Work out the finished part from the listing and answer in its coordinate system (mm). A direction names the side the tool comes from. Round coordinates to 2 decimals unless told otherwise and drop trailing zeros. Order: outer loops, then holes, each group sorted by start corner. A loop starts at its lowest first (then second) coordinate and runs counter-clockwise, first axis right, second up.
from build123d import *

# Parameters (mm, degrees)
SKETCH_2_W           = 30.5
SKETCH_2_H           = 20.5
SKETCH_2_W_2         = 22.5
SKETCH_2_H_2         = 12.5
EXTRUDE_1_DEPTH      = 12
SKETCH_3_W           = 2.75
SKETCH_3_H           = 10
EXTRUDE_2_DEPTH      = 3
SKETCH_4_W           = 4.940698383
SKETCH_4_H           = 10
CUT_EXTRUDE_1_DEPTH  = 9
SKETCH_7_R           = 1.25
CUT_EXTRUDE_2_DEPTH  = 23.584563312
SKETCH_12_W          = 15
SKETCH_12_H          = 20.5
EXTRUDE_5_DEPTH      = 15
SKETCH_13_W          = 10
SKETCH_13_H          = 10
CUT_EXTRUDE_6_DEPTH  = 12
EXTRUDE_7_REACH      = 33.133
SKETCH_15_R          = 1.5
CUT_EXTRUDE_7_DEPTH  = 32.30994251
SKETCH_16_W          = 10.43035396
SKETCH_16_H          = 7
CUT_EXTRUDE_8_DEPTH  = 23
CUT_EXTRUDE_9_REACH  = 36.03
SKETCH_17_W          = 10.8
SKETCH_17_H          = 10.8
CUT_EXTRUDE_10_REACH = 33.31
SKETCH_19_W          = 22.9
SKETCH_19_H          = 13.3
CUT_EXTRUDE_12_DEPTH = 12


with BuildPart() as part:
    # 草图2 → 凸台-拉伸1 (new body)
    with BuildSketch(Plane.XY):
        Rectangle(SKETCH_2_W, SKETCH_2_H)
        Rectangle(SKETCH_2_W_2, SKETCH_2_H_2, mode=Mode.SUBTRACT)
    extrude(amount=EXTRUDE_1_DEPTH)

    # 草图3 → 凸台-拉伸2 (add)
    with BuildSketch(Plane.XY.offset(12)):
        with Locations((-16.625, 0)):
            Rectangle(SKETCH_3_W, SKETCH_3_H)
    extrude_2 = extrude(amount=-EXTRUDE_2_DEPTH)

    # 镜向1: 凸台-拉伸2 across plane
    add(extrude_2.mirror(Plane(origin=(0, 0, 0), x_dir=(0, 0, 1), z_dir=(1, 0, 0))))

    # 草图4 → 切除-拉伸1 (cut)
    with BuildSketch(Plane(origin=(0, 0, 0), x_dir=(-1, 0, 0), z_dir=(0, 0, -1))):
        with Locations((15.220349192, 0)):
            Rectangle(SKETCH_4_W, SKETCH_4_H)
    cut_extrude_1 = extrude(amount=-CUT_EXTRUDE_1_DEPTH, mode=Mode.SUBTRACT)

    # 镜向2: 切除-拉伸1 across plane
    add(cut_extrude_1.mirror(Plane(origin=(0, 0, 0), x_dir=(0, 0, 1), z_dir=(1, 0, 0))), mode=Mode.SUBTRACT)

    # 草图7 → 切除-拉伸2 (cut, through all)
    with BuildSketch(Plane(origin=(0, 0, 9), x_dir=(-1, 0, 0), z_dir=(0, 0, -1))):
        with Locations((15.25, 0)):
            Circle(SKETCH_7_R)
    extrude(amount=-CUT_EXTRUDE_2_DEPTH, mode=Mode.SUBTRACT)

    # 草图12 → 凸台-拉伸5 (add)
    with BuildSketch(Plane(origin=(0, 0, 0), x_dir=(-1, 0, 0), z_dir=(0, 0, -1))):
        Rectangle(SKETCH_12_W, SKETCH_12_H)
    extrude(amount=EXTRUDE_5_DEPTH)

    # 草图13 → 切除-拉伸6 (cut)
    with BuildSketch(Plane(origin=(0, 0, -15), x_dir=(-1, 0, 0), z_dir=(0, 0, -1))):
        Rectangle(SKETCH_13_W, SKETCH_13_H)
    extrude(amount=-CUT_EXTRUDE_6_DEPTH, mode=Mode.SUBTRACT)

    # 凸台-拉伸7: up to this face of the body (flat: up to its plane)
    extrude_7_end = Plane(part.part.faces().sort_by_distance((0, 10.25, 0.860406091))[0])
    # 草图14 → 凸台-拉伸7 (add, up to the picked face)
    with BuildSketch(Plane.XZ.offset(10.25), mode=Mode.PRIVATE) as extrude_7_sk1:
        Polygon((-7.5, -3.75), (-7.5, 0), (-12.905079067, 0), align=None)
    extrude_7_tool1 = split(extrude(extrude_7_sk1.sketch, amount=-EXTRUDE_7_REACH, mode=Mode.PRIVATE), bisect_by=extrude_7_end, keep=Keep.BOTH, mode=Mode.PRIVATE)
    extrude_7 = extrude_7_tool1.solids().sort_by(Axis((-9.301693, -10.25, -1.25), (0, 1, 0)))[0]
    add(extrude_7)

    # 镜向6: 凸台-拉伸7 across plane
    add(extrude_7.mirror(Plane(origin=(0, 0, 0), x_dir=(0, 0, 1), z_dir=(1, 0, 0))))

    # 草图15 → 切除-拉伸7 (cut, through all)
    with BuildSketch(Plane.ZY.offset(7.5)):
        with Locations((-11, 0)):
            Circle(SKETCH_15_R)
    extrude(amount=-CUT_EXTRUDE_7_DEPTH, mode=Mode.SUBTRACT)

    # 草图16 → 切除-拉伸8 (cut)
    with BuildSketch(Plane.XY):
        with Locations((16.46517698, 0)):
            Rectangle(SKETCH_16_W, SKETCH_16_H)
    extrude(amount=CUT_EXTRUDE_8_DEPTH, mode=Mode.SUBTRACT)

    # 草图17 → 切除-拉伸9 (cut, up to next)
    with BuildSketch(Plane(origin=(0, 0, -15), x_dir=(-1, 0, 0), z_dir=(0, 0, -1)), mode=Mode.PRIVATE) as cut_extrude_9_sk1:
        Rectangle(SKETCH_17_W, SKETCH_17_H)
    cut_extrude_9_tool1 = extrude(cut_extrude_9_sk1.sketch, amount=-CUT_EXTRUDE_9_REACH, mode=Mode.PRIVATE) & part.part
    add(cut_extrude_9_tool1.solids().sort_by_distance((0, 0, -15))[0], mode=Mode.SUBTRACT)

    # 草图18 → 切除-拉伸10 (cut, up to next)
    with BuildSketch(Plane.ZY.offset(7.5), mode=Mode.PRIVATE) as cut_extrude_10_sk1:
        Polygon((-9.267949192, 3), (-12.732050808, 3), (-14.464101615, 0), (-12.732050808, -3), (-9.267949192, -3), (-7.535898385, 0), align=None)
    cut_extrude_10_tool1 = extrude(cut_extrude_10_sk1.sketch, amount=-CUT_EXTRUDE_10_REACH, mode=Mode.PRIVATE) & part.part
    add(cut_extrude_10_tool1.solids().sort_by_distance((-7.5, 0, -11))[0], mode=Mode.SUBTRACT)

    # 草图19 → 切除-拉伸12 (cut)
    with BuildSketch(Plane.XY.offset(12)):
        with Locations((-0.2, 0)):
            Rectangle(SKETCH_19_W, SKETCH_19_H)
    extrude(amount=-CUT_EXTRUDE_12_DEPTH, mode=Mode.SUBTRACT)


solid = part.part
Item 1: Given pin 1 (1 mm diameter, centred on y = -7, z = 6, fed in from -X); pin 2 (9 mm diameter, centred on y = 3.5, z = -10.5, fed in from -X); pin 3 (3.5 mm diameter, centred on y = -1, z = 4, fed in from +X), each flat-ended and moving along its own axis, determine where each tip first touches the part or whether it passes through.
Item 2: For a pull along X with two mould halves and no side action, classify faces 5 (the face through (0, -5.4, -8)), 6 (the face through (15.25, -8, 6)), 7 (the face through (-7.5, 0, -7)) as released by +X, released by -X, zero draft, split by the parting line, or undercut.
Item 3: Find the intervals of material crossed by line 1 along X through (y, z) = (4.5, 3.25); line 2 along Y through (x, z) = (3.5, -5.5); line 3 along Y through (x, z) = (6, 9.25), in increasing order.
Item 4: Find section C-C (y = 8.5). Write down the section's boundary in (x, z), plus the area to 3 significant figures.
Item 5: Find section A-A (z = -11). Write down the section's boundary in (x, y).
Item 6: Find section B-B (x = 0.5). Write down the section's boundary in (y, z).
Item 7: A tool of negligible diameter and unlimited length cuts with its end or side. For faces 1 (the face through (-5.4, 0, -6)), 2 (the face through (-6, -3, -11)), 3 (the face through (14, -8, 0)), 4 (the face through (17, -5, 11)), from which of +Z, -Z, +X, -X, +Y, -Y can it reach the whole face along a straight path? Write none if from no direction.
Item 8: Find section D-D (x = -7). Write down the section's boundary in (y, z).
Model answer:
1. pin 1: stops at x = -15.25
1. pin 2: stops at x = -7.5
1. pin 3: stops at x = -11.65
2. face 5: undercut
2. face 6: released by +X
2. face 7: released by -X
3. line 1: x = -12.75 to -11.65, 11.25 to 12.75
3. line 2: y = -10.25 to -5.4, 5.4 to 10.25
3. line 3: y = -10.25 to -6.65, 6.65 to 10.25
4. outline: (-15.25, 0) - (-12.91, 0) - (-7.5, -3.75) - (-7.5, -15) - (7.5, -15) - (7.5, -3.75) - (12.91, 0) - (15.25, 0) - (15.25, 12) - (-15.25, 12) - close
4. area: 611 mm2
5. outline: (-7.5, -10.25) - (7.5, -10.25) - (7.5, -1.5) - (5.4, -1.5) - (5.4, -5.4) - (-5.4, -5.4) - (-5.4, -3) - (-7.5, -3) - close; (-7.5, 3) - (-5.4, 3) - (-5.4, 5.4) - (5.4, 5.4) - (5.4, 1.5) - (7.5, 1.5) - (7.5, 10.25) - (-7.5, 10.25) - close
6. outline: (-10.25, -15) - (-5.4, -15) - (-5.4, 0) - (-6.65, 0) - (-6.65, 12) - (-10.25, 12) - close; (5.4, -15) - (10.25, -15) - (10.25, 12) - (6.65, 12) - (6.65, 0) - (5.4, 0) - close
7. face 1: +Z, -Z
7. face 2: -X
7. face 3: -Z, +X, +Y, -Y
7. face 4: +Z, -Z, +X, -Y
8. outline: (-10.25, -15) - (10.25, -15) - (10.25, 12) - (6.65, 12) - (6.65, 0) - (-6.65, 0) - (-6.65, 12) - (-10.25, 12) - close; hole (-3, -12.73) - (0, -14.46) - (3, -12.73) - (3, -9.27) - (0, -7.54) - (-3, -9.27) - close
